The model under review builds one solid part; all positions refer to its coordinate system, in mm. A direction names the side the tool comes from. Coordinates: 2 decimals unless noted, no trailing zeros. Order: outer loops, then holes, each group sorted by start corner. A loop starts at its lowest first (then second) coordinate and runs counter-clockwise, first axis right, second up.
from build123d import *

# Parameters (mm, degrees)
SKETCH1_R           = 3.302
BOSS_EXTRUDE1_DEPTH = 9.525
FILLET1_R           = 6.35
SKETCH2_R           = 2.286
CUT_EXTRUDE1_DEPTH  = 38.162422217
BOSS_EXTRUDE2_START = 9.525
SKETCH3_R           = 6.35
SKETCH3_R_2         = 3.302
BOSS_EXTRUDE2_DEPTH = 9.525


with BuildPart() as part:
    # Sketch1 → Boss-Extrude1 (new body)
    with BuildSketch(Plane(origin=(0, 0, 0), x_dir=(1, 0, 0), z_dir=(0, 1, 0))):
        with BuildLine():
            Line((-12.7, -12.7), (12.7, -12.7))
            Line((12.7, -12.7), (22.86, -5.08))
            ThreePointArc((22.86, -5.08), (25.4, 0), (22.86, 5.08))
            Line((22.86, 5.08), (12.7, 12.7))
            Line((12.7, 12.7), (-12.7, 12.7))
            Line((-12.7, 12.7), (-22.86, 5.08))
            ThreePointArc((-22.86, 5.08), (-25.4, 0), (-22.86, -5.08))
            Line((-22.86, -5.08), (-12.7, -12.7))
        make_face()
        with Locations(Location((-19.05, 0, 0), (0, 0, 90))):
            Circle(SKETCH1_R, mode=Mode.SUBTRACT)
        with Locations(Location((19.05, 0, 0), (0, 0, 90))):
            Circle(SKETCH1_R, mode=Mode.SUBTRACT)
        with BuildLine():
            Line((4.7625, -10.1854), (8.329805012, -10.1854))
            Line((8.329805012, -10.1854), (8.376905012, -10.154))
            Line((8.376905012, -10.154), (9.416515139, -10.154))
            ThreePointArc((9.416515139, -10.154), (9.501675056, -10.1507417), (9.586332782, -10.140948982))
            Line((9.586332782, -10.140948982), (9.615351798, -10.140948982))
            ThreePointArc((9.615351798, -10.140948982), (10.251622353, -9.784337345), (10.504, -9.1))
            Line((10.504, -9.1), (10.504, -8.735936675))
            Line((10.504, -8.735936675), (11.2014, -8.271003341))
            Line((11.2014, -8.271003341), (11.2014, 8.271003341))
            Line((11.2014, 8.271003341), (8.329805012, 10.1854))
            Line((8.329805012, 10.1854), (4.7625, 10.1854))
            Line((4.7625, 10.1854), (4.7625, 10.4394))
            Line((4.7625, 10.4394), (-4.7625, 10.4394))
            Line((-4.7625, 10.4394), (-4.7625, 10.1854))
            Line((-4.7625, 10.1854), (-8.329805012, 10.1854))
            Line((-8.329805012, 10.1854), (-11.2014, 8.271003341))
            Line((-11.2014, 8.271003341), (-11.2014, -8.271003341))
            Line((-11.2014, -8.271003341), (-10.504, -8.735936675))
            Line((-10.504, -8.735936675), (-10.504, -9.1))
            ThreePointArc((-10.504, -9.1), (-10.251622353, -9.784337345), (-9.615351798, -10.140948982))
            Line((-9.615351798, -10.140948982), (-9.586332782, -10.140948982))
            ThreePointArc((-9.586332782, -10.140948982), (-9.501675056, -10.1507417), (-9.416515139, -10.154))
            Line((-9.416515139, -10.154), (-8.376905012, -10.154))
            Line((-8.376905012, -10.154), (-8.329805012, -10.1854))
            Line((-8.329805012, -10.1854), (-4.7625, -10.1854))
            Line((-4.7625, -10.1854), (-4.7625, -10.4394))
            Line((-4.7625, -10.4394), (4.7625, -10.4394))
            Line((4.7625, -10.4394), (4.7625, -10.1854))
        make_face(mode=Mode.SUBTRACT)
    extrude(amount=BOSS_EXTRUDE1_DEPTH)

    # Fillet1
    fillet1_edges = [part.edges().sort_by_distance(p)[0] for p in [
        (12.7, 4.7625, -12.7),
        (12.7, 4.7625, 12.7),
        (-12.7, 4.7625, 12.7),
        (-12.7, 4.7625, -12.7),
    ]]
    fillet(fillet1_edges, radius=FILLET1_R)

    # Sketch2 → Cut-Extrude1 (cut, through all)
    with BuildSketch(Plane.XY.offset(12.7)):
        with Locations((0, 4.7625)):
            Circle(SKETCH2_R)
    extrude(amount=-CUT_EXTRUDE1_DEPTH, mode=Mode.SUBTRACT)

    # Sketch3 → Boss-Extrude2 (add)
    # profile 1 of 2: a face of its own
    with BuildSketch(Plane(origin=(0, 0, 0), x_dir=(-1, 0, 0), z_dir=(0, -1, 0)).offset(BOSS_EXTRUDE2_START)):
        with Locations(Location((19.05, 0, 0), (0, 0, 90))):
            Circle(SKETCH3_R)
        with Locations(Location((19.05, 0, 0), (0, 0, 90))):
            Circle(SKETCH3_R_2, mode=Mode.SUBTRACT)
    # profile 2 of 2: a face of its own
    with BuildSketch(Plane(origin=(0, 0, 0), x_dir=(-1, 0, 0), z_dir=(0, -1, 0)).offset(BOSS_EXTRUDE2_START)):
        with Locations(Location((-19.05, 0, 0), (0, 0, 90))):
            Circle(SKETCH3_R)
        with Locations(Location((-19.05, 0, 0), (0, 0, 90))):
            Circle(SKETCH3_R_2, mode=Mode.SUBTRACT)
    extrude(amount=-BOSS_EXTRUDE2_DEPTH)


solid = part.part
(1) Consider section B-B (x = 0). Give the boundary of the cut face in (y, z) (1 decimal).
(2) Consider section C-C (z = 0). Give the boundary of the cut face in (x, y) (3 decimals), then the cut area to 3 significant figures.
(3) The part is to be moulded in two halves that separate along Y. For faces 3 (the face through (7, 5, 10.185)), 4 (the face through (-12, 9.525, 0)), 5 (the face through (16, -9.525, -3)), 6 (the face through (-0.5, 2.53, 11.59)), say which applies: +Y half, -Y half, draft (parallel to the pull), parting line (faces both ways), or undercut.
(4) Insertion check: pin 1 Ø1 at (x, y) = (19.5, 5.5) entering from -Z (3 decimals); pin 2 Ø3 at (y, z) = (-2, -3) entering from +X; pin 3 Ø12 at (x, z) = (-0.5, -5.5) entering from -Y. Each pin has a flat end and moves straight along its axis. Give the tip position at first contact, or say it passes through.
(5) Tool access review of faces 1 (the face through (18.567, 4.696, 8.299)), 2 (the face through (2.2, 3.6, -10.439)): name each direction out of +Z, -Z, +X, -X, +Y, -Y from which nothing blocks a thin tool from reaching the whole face with its end or side.
(6) Consider section A-A (z = -7). Give the boundary of the cut face in (x, y) (3 decimals), then the cut area to 3 significant figures.
(7) Consider section D-D (y = -3.75). Give the boundary of the cut face in (x, z), then the cut area to 3 significant figures.
(8) Wall thickness on line 1 (X direction, y = -2, z = 0); line 2 (Z direction, x = -6.5, y = 3.25); line 3 (Z direction, x = -19.05, y = -7): over which ranges is each line inside the solid? List them lowest first.
Findings:
1. outline: (0, -12.7) - (2.5, -12.7) - (2.5, -10.4) - (0, -10.4) - close; (0, 10.4) - (2.5, 10.4) - (2.5, 12.7) - (0, 12.7) - close; (7, -12.7) - (9.5, -12.7) - (9.5, -10.4) - (7, -10.4) - close; (7, 10.4) - (9.5, 10.4) - (9.5, 12.7) - (7, 12.7) - close
2. outline: (-25.4, -9.525) - (-22.352, -9.525) - (-22.352, 9.525) - (-25.4, 9.525) - close; (-15.748, -9.525) - (-12.7, -9.525) - (-12.7, 0) - (-11.201, 0) - (-11.201, 9.525) - (-15.748, 9.525) - close; (11.201, 0) - (12.7, 0) - (12.7, -9.525) - (15.748, -9.525) - (15.748, 9.525) - (11.201, 9.525) - close; (22.352, -9.525) - (25.4, -9.525) - (25.4, 9.525) - (22.352, 9.525) - close
2. area: 261 mm2
3. face 3: draft
3. face 4: +Y half
3. face 5: -Y half
3. face 6: undercut
4. pin 1: stops at z = -7.975
4. pin 2: stops at x = 25.22
4. pin 3: stops at y = 0
5. face 1: +Z, +X, +Y, -Y
5. face 2: +Y, -Y
6. outline: (-20.3, 0) - (-11.201, 0) - (-11.201, 9.525) - (-20.3, 9.525) - close; (11.201, 0) - (20.3, 0) - (20.3, 9.525) - (11.201, 9.525) - close
6. area: 173 mm2
7. outline: circle Ø12.7 at (-19.05, 0); circle Ø12.7 at (19.05, 0); hole circle Ø6.6 at (-19.05, 0); hole circle Ø6.6 at (19.05, 0)
7. area: 185 mm2
8. line 1: x = -25.4 to -22.35, -15.75 to -12.7, 12.7 to 15.75, 22.35 to 25.4
8. line 2: z = -12.7 to -10.19, 10.19 to 12.7
8. line 3: z = -6.35 to -3.3, 3.3 to 6.35
